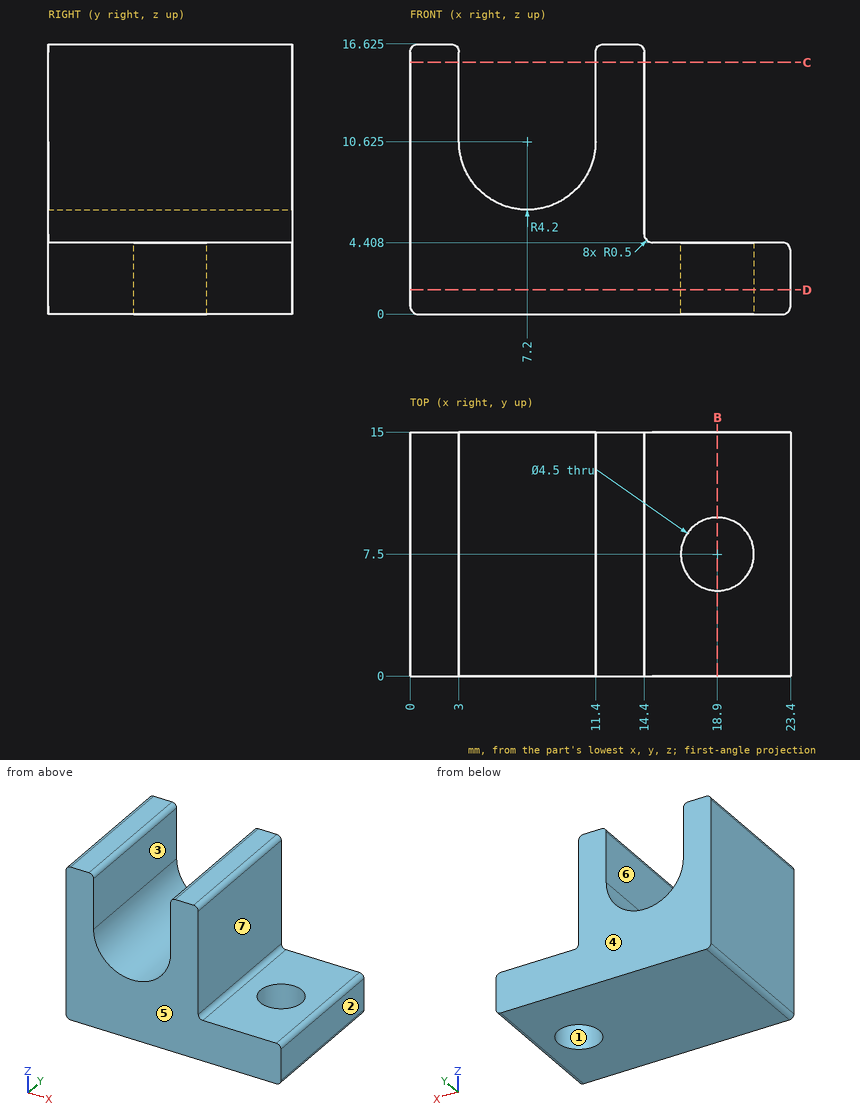
The drawing under review shows one solid part. Ordinate dimensions are in mm from its lowest x, y, z. A direction names the side the tool comes from. Round coordinates to 2 decimals unless told otherwise and drop trailing zeros. Loops run counter-clockwise (first coordinate to the right, second up) from the corner with the lowest first, then second, coordinate; pieces in that order, holes last. Notation, with made-up numbers: (46, 28.5) - (88, 28.5) arc R24 ccw to (88, 52.5) - close; hole circle Ø11 at (41.5, 68.5). An arc over 180 degrees is marked (long way). One line per item, written item: value. Start each with the question number.
1) Insertion check: pin 1 Ø1.5 at (x, y) = (18.5, 4) entering from +Z; pin 2 Ø3.5 at (y, z) = (5, 9) entering from +X. Each pin has a flat end and moves straight along its axis. Give the tip position at first contact, or say it passes through.
2) Consider section C-C on z = 15.5. Give the boundary of the cut face in (x, y).
3) Draft analysis for pull direction X (two halves, no side actions). For the marked faces 1, 2, 3 and 4, state which applies: +X half, -X half, draft (parallel to the pull), parting line (faces both ways), or undercut.
4) To check wall thickness, follow L1, parallel to Y at x = 18.9, z = 1.1; L2, parallel to X at y = 12.5, z = 14.5; L3, parallel to Z at x = 20.25, y = 10.5. State the ranges of each line that lie inside material, in increasing order. Write a range as from..to.
5) Consider section D-D on z = 1.5. Give the boundary of the cut face in (x, y), then the cut area to 3 significant figures.
6) For the marked faces 5, 6 and 7, list the 3-axis set-ups (+Z, -Z, +X, -X, +Y, -Y) from which the entire face can be reached by the end or side of a thin tool; tool diameter is ignored.
7) Consider section B-B on x = 18.9. Give the boundary of the cut face in (y, z).
Reported:
1. pin 1: stops at z = 4.41
1. pin 2: stops at x = 14.4
2. outline: (0, 0) - (3, 0) - (3, 15) - (0, 15) - close; (11.4, 0) - (14.4, 0) - (14.4, 15) - (11.4, 15) - close
3. face 1: undercut
3. face 2: +X half
3. face 3: undercut
3. face 4: draft
4. L1: y = 0..5.25, 9.75..15
4. L2: x = 0..3, 11.4..14.4
4. L3: z = 0..4.41
5. outline: (0, 0) - (23.4, 0) - (23.4, 15) - (0, 15) - close; hole circle Ø4.5 at (18.9, 7.5)
5. area: 335 mm^2
6. face 5: +Z, -Z, +X, -X, -Y
6. face 6: +Z, +Y, -Y
6. face 7: +Z, +X, +Y, -Y
7. outline: (0, 0) - (5.25, 0) - (5.25, 4.41) - (0, 4.41) - close; (9.75, 0) - (15, 0) - (15, 4.41) - (9.75, 4.41) - close
